```python
from build123d import *

# Parameters (mm, degrees)
SKETCH1_R            = 200
BOSS_EXTRUDE1_DEPTH  = 100
BOSS_EXTRUDE1_TAPER  = 14
SKETCH2_R            = 10
BOSS_EXTRUDE2_DEPTH  = 400
SKETCH7_W            = 480
SKETCH7_H            = 500
BOSS_EXTRUDE8_DEPTH  = 50
SKETCH8_W            = 480
SKETCH8_H            = 20
BOSS_EXTRUDE9_DEPTH  = 750
SKETCH9_W            = 20
SKETCH9_H            = 480
BOSS_EXTRUDE10_DEPTH = 250


with BuildPart() as part:
    # Sketch1 → Boss-Extrude1 (new body)
    with BuildSketch(Plane(origin=(0, 0, 0), x_dir=(1, 0, 0), z_dir=(0, 1, 0))):
        Circle(SKETCH1_R)
    extrude(amount=BOSS_EXTRUDE1_DEPTH, taper=BOSS_EXTRUDE1_TAPER)

    # Sketch2 → Boss-Extrude2 (add)
    with BuildSketch(Plane(origin=(0, 100, 0), x_dir=(1, 0, 0), z_dir=(0, 1, 0))):
        with Locations(Location((86.344755042, 0, 0), (0, 0, 270))):
            Circle(SKETCH2_R)
        with Locations(Location((0, -86.344755042, 0), (0, 0, 270))):
            Circle(SKETCH2_R)
        with Locations(Location((-86.344755042, 0, 0), (0, 0, 270))):
            Circle(SKETCH2_R)
        with Locations(Location((0, 86.344755042, 0), (0, 0, 270))):
            Circle(SKETCH2_R)
    extrude(amount=BOSS_EXTRUDE2_DEPTH)

    # Sketch7 → Boss-Extrude8 (add)
    with BuildSketch(Plane(origin=(0, 500, 0), x_dir=(1, 0, 0), z_dir=(0, 1, 0))):
        Rectangle(SKETCH7_W, SKETCH7_H)
    extrude(amount=BOSS_EXTRUDE8_DEPTH)

    # Sketch8 → Boss-Extrude9 (add)
    with BuildSketch(Plane(origin=(0, 550, 0), x_dir=(1, 0, 0), z_dir=(0, 1, 0))):
        with Locations((0, 240)):
            Rectangle(SKETCH8_W, SKETCH8_H)
    extrude(amount=BOSS_EXTRUDE9_DEPTH)

    # Sketch9 → Boss-Extrude10 (add)
    with BuildSketch(Plane(origin=(0, 550, 0), x_dir=(1, 0, 0), z_dir=(0, 1, 0))):
        with Locations((-230, -10)):
            Rectangle(SKETCH9_W, SKETCH9_H)
        with Locations((230, -10)):
            Rectangle(SKETCH9_W, SKETCH9_H)
    extrude(amount=BOSS_EXTRUDE10_DEPTH)


solid = part.part
```
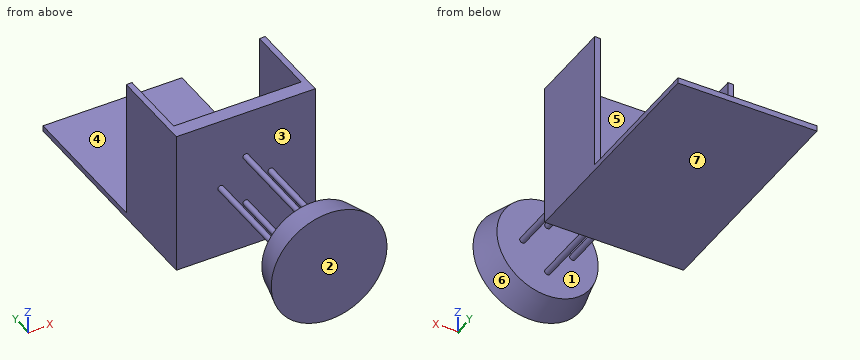
Could you check a few things on this model? Use its own coordinates, in mm. Face numbers are marked on the shaded views. A direction names the side the tool comes from. Round coordinates to 2 decimals unless told otherwise and drop trailing zeros. Loops run counter-clockwise (first coordinate to the right, second up) from the corner with the lowest first, then second, coordinate; pieces in that order, holes last. Notation, with made-up numbers: (-32, 67.25) - (11, 67.25) arc R26 cw to (11, 84.25) - close; hole circle Ø10 at (79, 21.25). An arc over 180 degrees is marked (long way). Answer in a Markdown table with one row per item. Add a question column.
(1) I need wall thicknesses on line 1 along Y through (x, z) = (32, 33); line 2 along X through (y, z) = (603, 223); line 3 along Z through (x, y) = (-38, 751). Which ranges of each line are inside material? Lowest first, please.
(2) For the marked faces 5, 6 and 7, which set-ups out of +Z, -Z, +X, -X, +Y, -Y let a thin tool reach every point of the face, with its end or its side?
(3) If we section it at A-A (y = 566): Please give me the cut outline in (x, z), plus the area to 3 significant figures.
(4) If we mould it in two halves opening along Y, with no side actions, what happens to the marked faces 1, 2, 3 and 4? For each: pulls with the +Y half, pulls with the -Y half, needs draft (parallel to the pull), parting line crosses it, or undercut.
(5) I'm going to push flat-ended pins straight in: pin 1 (4 mm diameter, centred on x = 98, z = 109, fed in from +Y); pin 2 (10 mm diameter, centred on x = 231, z = 110, fed in from +Y). Where does each tip first touch, or does it pass through?
Model answer:
| question | item | result |
|---|---|---|
| 1 | line 1 | y = 0 to 100, 500 to 550 |
| 1 | line 2 | x = -240 to -220, 220 to 240 |
| 1 | line 3 | z = -250 to -230 |
| 2 | face 5 | +Z, +Y |
| 2 | face 6 | none |
| 2 | face 7 | -Z, +X, -X, +Y, -Y |
| 3 | outline | (-240, -250) - (240, -250) - (240, 250) - (220, 250) - (220, -230) - (-220, -230) - (-220, 250) - (-240, 250) - close |
| 3 | area | 28,800 mm² |
| 4 | face 1 | undercut |
| 4 | face 2 | pulls with the -Y half |
| 4 | face 3 | undercut |
| 4 | face 4 | needs draft |
| 5 | pin 1 | stops at y = 550 |
| 5 | pin 2 | stops at y = 800 |
